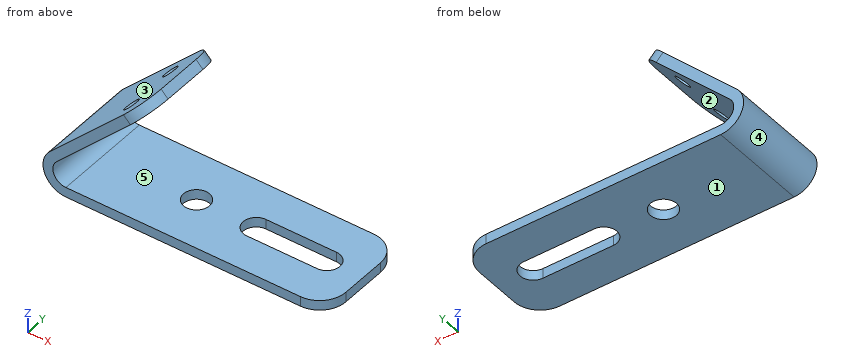
from build123d import *

# Parameters (mm, degrees)
F1_DEPTH = 19.05
F2_R     = 1.5
F3_DEPTH = 1.9
F4_R     = 2.5
F5_DEPTH = 25
F6_R     = 5


with BuildPart() as f1:
    # F0 (on Front) → F1 (new body)
    with BuildSketch(Plane.XZ):
        with BuildLine():
            Line((-50, 0), (0, 0))
            Line((0, 0), (0, 1.9))
            Line((0, 1.9), (-50, 1.9))
            ThreePointArc((-50, 1.9), (-52.3096988313, 3.4432914191), (-51.767766953, 6.167766953))
            Line((-51.767766953, 6.167766953), (-34.0900974233, 23.8454364826))
            Line((-34.0900974233, 23.8454364826), (-35.4336003076, 25.1889393669))
            Line((-35.4336003076, 25.1889393669), (-53.1112698372, 7.5112698372))
            ThreePointArc((-53.1112698372, 7.5112698372), (-54.065069943, 2.7161928976), (-50, 0))
        make_face()
    extrude(amount=-F1_DEPTH)

    # F2 (on face) → F3 (cut, through all)
    with BuildSketch(Plane(origin=(-30.3112698372, 0, 30.3112698372), x_dir=(0, -1, 0), z_dir=(-0.7071067812, 0, 0.7071067812))):
        with Locations((-14.55, -14.7440692221)):
            Circle(F2_R)
        with Locations((-4.5, -14.7440692221)):
            Circle(F2_R)
    extrude(amount=-F3_DEPTH, mode=Mode.SUBTRACT)

    # F4 (on face) → F5 (cut)
    with BuildSketch(Plane.XY.offset(1.9)):
        with BuildLine():
            Line((-7, 12.05), (-20.5371917859, 12.05))
            ThreePointArc((-20.5371917859, 12.05), (-23.0371917859, 9.55), (-20.5371917859, 7.05))
            Line((-20.5371917859, 7.05), (-7, 7.05))
            ThreePointArc((-7, 7.05), (-4.5, 9.55), (-7, 12.05))
        make_face()
        with Locations((-32, 9.55)):
            Circle(F4_R)
    extrude(amount=-F5_DEPTH, mode=Mode.SUBTRACT)

    # F6
    f6_edges = [f1.edges().sort_by_distance(p)[0] for p in [
        (-34.761849, 0, 24.517188),
        (0, 0, 0.95),
        (-34.761849, 19.05, 24.517188),
        (0, 19.05, 0.95),
    ]]
    fillet(f6_edges, radius=F6_R)


solid = f1.part
Can you work these out from the model? Positions are in its coordinate system, mm. Face numbers are marked on the shaded views. A direction names the side the tool comes from. Give positions to 0.01 mm unless a question says otherwise; leave off trailing zeros. Write each loop counter-clockwise with the first axis right and the second up, starting at its lowest first coordinate (ties: lowest second). Pieces come first, ordered by that corner, then holes. Notation, with made-up numbers: M -8,49 L 38,49 A20 cw 38,79 Z; hole C 69.25,87 d7. An arc over 180 degrees is marked long. Answer in a Markdown table with one row per item. Add a question column.
Item 1: Imagine slicing it at D-D, the plane z = 2.75. Write out the boundary of the cut face in (x, y).
Item 2: For pin 1 Ø3 at (y, z) = (3.5, 4) entering from +X; pin 2 Ø6 at (x, y) = (-29, 5) entering from +Z; pin 3 Ø6.5 at (x, y) = (-32, 9.55) entering from +Z, each with a flat end and sliding along its axis, tell me the tip position at first contact or that it passes through.
Item 3: Imagine slicing it at B-B, the plane y = 9.55. Write out the boundary of the cut face in (x, z).
Item 4: We'd pull the mould along Z, two halves only. Please class the marked faces 3, 4 and 5: released by +Z, released by -Z, zero draft, split by the parting line, or undercut.
Item 5: Please list where these lines run through material, in increasing order: L1, parallel to Y at x = -32, z = 0.8; L2, parallel to X at y = 11.25, z = 1.75; L3, parallel to Z at x = -29, y = 6.
Item 6: Imagine slicing it at A-A, the plane x = -32. Write out the boundary of the cut face in (y, z), plus the area to 3 significant figures.
Item 7: On a 3-axis mill with a long thin cutter (end or side, diameter ignored), from which of +Z, -Z, +X, -X, +Y, -Y can I reach the whole of each face in a straight line? I mean the marked faces 1 and 2. Say none if no direction works.
Item 8: Imagine slicing it at C-C, the plane x = -40. State how many separate pieces and enclosed holes the cut face has, plus the area to 3 significant figures.
Evaluation:
| question | item | result |
|---|---|---|
| 1 | outline | M -54.08,0 L -51.88,0 L -51.88,19.05 L -54.08,19.05 Z |
| 2 | pin 1 | stops at x = -51.62 |
| 2 | pin 2 | stops at z = 1.9 |
| 2 | pin 3 | stops at z = 25.01 |
| 3 | outline | M -53.11,7.51 A4.4 ccw -50,0 L -34.5,0 L -34.5,1.9 L -50,1.9 A2.5 cw -51.77,6.17 L -34.09,23.85 L -35.43,25.19 Z; M -29.5,0 L -23.04,0 L -23.04,1.9 L -29.5,1.9 Z; M -4.5,0 L 0,0 L 0,1.9 L -4.5,1.9 Z |
| 4 | face 3 | released by +Z |
| 4 | face 4 | split by the parting line |
| 4 | face 5 | undercut |
| 5 | L1 | y = 0 to 7.05, 12.05 to 19.05 |
| 5 | L2 | x = -53.51 to -33.83, -30.17 to -22.37, -5.17 to 0 |
| 5 | L3 | z = 0 to 1.9 |
| 6 | outline | M 0,0 L 7.05,0 L 7.05,1.9 L 0,1.9 Z; M 12.05,0 L 19.05,0 L 19.05,1.9 L 12.05,1.9 Z |
| 6 | area | 26.7 mm² |
| 7 | face 1 | -Z, +X, -X, +Y, -Y |
| 7 | face 2 | +X, +Y, -Y |
| 8 | separate pieces | 4 |
| 8 | enclosed holes | 0 |
| 8 | area | 72.5 mm² |
